```python
from build123d import *

# Parameters (mm, degrees)
F1_DEPTH = 90
F0_R     = 3
F2_DEPTH = 45


with BuildPart() as f1:
    # F0 (on Top) → F1 (new body)
    with BuildSketch(Plane.XY):
        with BuildLine():
            ThreePointArc((6.324555, 3), (6.829051, 1.537549), (7, 0))
            ThreePointArc((7, 0), (6.829051, -1.537549), (6.324555, -3))
            Line((6.324555, -3), (44.324555, -3))
            Line((44.324555, -3), (44.324555, 3))
            Line((44.324555, 3), (6.324555, 3))
        make_face()
    extrude(amount=F1_DEPTH)

    # F0 (on Top) → F2 (join)
    with BuildSketch(Plane.XY):
        with BuildLine():
            ThreePointArc((6.324555, -3), (6.829051, -1.537549), (7, 0))
            ThreePointArc((7, 0), (6.829051, 1.537549), (6.324555, 3))
            ThreePointArc((6.324555, 3), (-7, 0), (6.324555, -3))
        make_face()
        Circle(F0_R, mode=Mode.SUBTRACT)
    extrude(amount=F2_DEPTH)


solid = f1.part
```
Can you work these out from the model? Positions are in its coordinate system, mm. A direction names the side the tool comes from. Give positions to 0.01 mm unless a question says otherwise; leave off trailing zeros. Order: outer loops, then holes, each group sorted by start corner. A loop starts at its lowest first (then second) coordinate and runs counter-clockwise, first axis right, second up. Notation, with made-up numbers: (13, 45) - (66, 45) arc R33 ccw to (66, 75) - close; hole circle Ø1 at (9.25, 33.5). An arc over 180 degrees is marked (long way). Use a Markdown table: item, result. Add a question column.
Q1. On a 3-axis mill with a long thin cutter (end or side, diameter ignored), from which of +Z, -Z, +X, -X, +Y, -Y can I reach the whole of each face in a straight line? I mean faces 1 (the flat face through (26, 3, 44)), 2 (the flat face through (13, 0, 0)), 3 (the flat face through (25, -3, 44)). Say none if no direction works.
Q2. If we section it at C-C on y = -1.25: Write out the boundary of the cut face in (x, z), plus the area to 3 significant figures.
Q3. I'm going to push flat-ended pins straight in: pin 1 (11.5 mm diameter, centred on x = 25.5, z = 64.5, fed in from -Y); pin 2 (3 mm diameter, centred on y = 5.5, z = 28.5, fed in from -X); pin 3 (6 mm diameter, centred on x = 23.5, z = 38.5, fed in from +Y). Where does each tip first touch, or does it pass through?
Q4. If we section it at A-A on x = 0: Write out the boundary of the cut face in (y, z), plus the area to 3 significant figures.
Q5. Please list where these lines run through material, in increasing order: line 1 along Y through (x, z) = (0, 28); line 2 along Y through (x, z) = (20, 45.5); line 3 along Z through (x, y) = (-4.5, -5).
Q6. If we mould it in two halves opening along X, with no side actions, what happens to faces 4 (the flat face through (44.325, 0, 44)), 5 (the flat face through (25, 0, 90)), 6 (the cylindrical face through (-3, 0, 22))? For each: released by +X, released by -X, zero draft, split by the parting line, or undercut.
Q7. If we section it at D-D on z = 56.5: Write out the boundary of the cut face in (x, y), plus the area to 3 significant figures.
Q8. If we section it at B-B on z = 39.5: Write out the boundary of the cut face in (x, y).
Answers follow:
| question | item | result |
|---|---|---|
| 1 | face 1 | +Z, -Z, +X, +Y |
| 1 | face 2 | -Z, +X, -X, +Y, -Y |
| 1 | face 3 | +Z, -Z, +X, -Y |
| 2 | outline | (-6.89, 0) - (-2.73, 0) - (-2.73, 45) - (-6.89, 45) - close; (2.73, 0) - (44.32, 0) - (44.32, 90) - (6.89, 90) - (6.89, 45) - (2.73, 45) - close |
| 2 | area | 3,740 mm^2 |
| 3 | pin 1 | stops at y = -3 |
| 3 | pin 2 | stops at x = -5.74 |
| 3 | pin 3 | stops at y = 3 |
| 4 | outline | (-7, 0) - (-3, 0) - (-3, 45) - (-7, 45) - close; (3, 0) - (7, 0) - (7, 45) - (3, 45) - close |
| 4 | area | 360 mm^2 |
| 5 | line 1 | y = -7 to -3, 3 to 7 |
| 5 | line 2 | y = -3 to 3 |
| 5 | line 3 | z = 0 to 45 |
| 6 | face 4 | released by +X |
| 6 | face 5 | zero draft |
| 6 | face 6 | undercut |
| 7 | outline | (6.32, -3) - (44.32, -3) - (44.32, 3) - (6.32, 3) arc R7 cw to (7, 0) arc R7 cw to start |
| 7 | area | 225 mm^2 |
| 8 | outline | (6.32, -3) - (44.32, -3) - (44.32, 3) - (6.32, 3) arc R7 ccw (long way) to start; hole circle Ø6 at (0, 0) |
